Source: CAD feature listing. Evaluate the final solid. Frame: model axes, mm. Face numbers are marked on the shaded views. A direction names the side the tool comes from. Round coordinates to 2 decimals unless told otherwise and drop trailing zeros. Write each loop counter-clockwise with the first axis right and the second up, starting at its lowest first coordinate (ties: lowest second). Pieces come first, ordered by that corner, then holes. Notation, with made-up numbers: M 61.25,31.25 L 104.25,31.25 A17 cw 104.25,64.25 Z; hole C 42,84 d2. An arc over 180 degrees is marked long. Use a Markdown table: item, result.
Autodesk Fusion 360 part; units mm, degrees
sketch "Sketch1" plane through (0, 0, 0) normal (0, 0, 1) x (1, 0, 0)
  line L0 (20.9846, 55.2598) -> (20.9846, 21.2598)
  line L1 (20.9846, 55.2598) -> (24.9846, 55.2598)
  line L2 (24.9846, 55.2598) -> (24.9846, 53.2598)
  line L3 (24.9846, 53.2598) -> (26.9846, 53.2598)
  line L4 (26.9846, 53.2598) -> (26.9846, 57.2598)
  line L5 (26.9846, 57.2598) -> (7.9846, 57.2598)
  line L6 (7.9846, 57.2598) -> (7.9846, 37.2598)
  line L7 (7.9846, 37.2598) -> (18.9846, 37.2598)
  line L8 (18.9846, 37.2598) -> (18.9846, 19.2598)
  line L9 (18.9846, 19.2598) -> (26.485, 19.2598)
  line L10 (20.9846, 21.2598) -> (24.6846, 21.2598)
  line L11 (24.6846, 21.2598) -> (25.485, 22.2598)
  line L12 (25.485, 22.2598) -> (26.485, 22.2598)
  line L13 (26.485, 22.2598) -> (26.485, 19.2598)
  line L14 (9.9846, 55.2598) -> (15.9742, 55.2598)
  line L15 (15.9742, 55.2598) -> (9.9846, 49.9357)
  line L16 (9.9846, 49.9357) -> (9.9846, 55.2598)
  line L17 (9.9846, 44.5839) -> (9.9846, 39.2598)
  line L18 (9.9846, 39.2598) -> (15.9742, 39.2598)
  line L19 (9.9846, 44.5839) -> (15.9742, 39.2598)
  line L20 (9.9846, 47.2598) -> (18.9846, 55.2598)
  line L21 (18.9846, 39.2598) -> (9.9846, 47.2598)
  line L22 (18.9846, 39.2598) -> (18.9846, 55.2598)
  dimension "d1" = 2
  dimension "d2" = 4
  dimension "d3" = 2
  dimension "d4" = 2
  dimension "d5" = 13
  dimension "d6" = 34
  dimension "d7" = 1
  dimension "d8" = 3.7
  dimension "d9" = 1
  dimension "d10" = 2
  dimension "d11" = 20
  dimension "d15" = 2
  dimension "d25" = 2
  dimension "d26" = 2
  dimension "d27" = 2
  dimension "d29" = 2
  dimension "d30" = 2
  dimension "d31" = 2
  dimension "d32" = 2
  dimension "d34" = 2
  dimension "d35" = 2
extrude "Extrude1" add sketch "Sketch1" along normal blind 7.7
fillet "Fillet1" radius 1 9 edges at (7.9846, 37.2598, 3.85) (18.9846, 37.2598, 3.85) (18.9846, 19.2598, 3.85) (26.485, 19.2598, 3.85) (7.9846, 57.2598, 3.85) (26.485, 22.2598, 3.85) (24.9846, 53.2598, 3.85) (26.9846, 53.2598, 3.85) (26.9846, 57.2598, 3.85)
fillet "Fillet1" radius 1 9 edges at (9.9846, 55.2598, 3.85) (15.9742, 55.2598, 3.85) (15.9742, 39.2598, 3.85) (9.9846, 39.2598, 3.85) (20.9846, 38.2598, 7.7) (9.9846, 49.9357, 3.85) (9.9846, 47.2598, 3.85) (18.9846, 55.2598, 3.85) (18.9846, 39.2598, 3.85)
sketch "Sketch2" plane through (0, 57.2598, 0) normal (0, 1, 0) x (-1, 0, 0)
  line L0 (-25.9846, 7.7) -> (-25.9846, 0)
  line L1 (-25.9846, 0) -> (-8.9846, 0)
  line L2 (-8.9846, 0) -> (-8.9846, 7.7)
  line L3 (-8.9846, 7.7) -> (-25.9846, 7.7)
  line L4 (-26.9846, 7.7) -> (-26.9846, 0)
  line L5 (-7.9846, 0) -> (-7.9846, 7.7)
  line L6 (-20.9846, 0) -> (-20.9846, 6.7)
  point P0 (-11.9846, 4)
  point P1 (-20.9846, 0)
  point P2 (-11.9846, 3.7)
  dimension "d16" = 4
  dimension "d22" = 9
  dimension "d23" = 9
  dimension "d24" = 4
hole "Hole1" at (11.9846, 57.2598, 4) at (11.9846, 57.2598, 3.7) direction (0, -1, 0) diameter 5 depth 18 tip angle 160
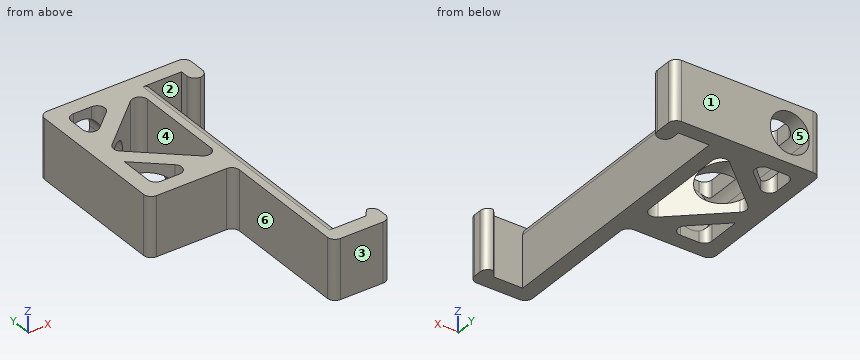
Q1. Section A-A on x = 24. Return loops of the section in (y, z).
Results are:
| item | result |
|---|---|
| outline | M 19.26,0 L 21.26,0 L 21.26,7.7 L 19.26,7.7 Z; M 55.26,0 L 57.26,0 L 57.26,7.7 L 55.26,7.7 Z |
Q2. Line query: L1, parallel to X at y = 53, z = 3; L2, parallel to Y at x = 22.5, z = 3.25; L3, parallel to X at y = 52, z = 0.75. Output: solid intervals per line, ascending.
Results are:
| item | result |
|---|---|
| L1 | 7.98 to 9.58, 14.38 to 16.44, 18.98 to 20.98 |
| L2 | 19.26 to 21.26, 55.26 to 57.26 |
| L3 | 7.98 to 10, 12.31 to 15.32, 18.98 to 20.98 |
Q3. Reachability of the marked faces 4, 5 and 6 from +Z, -Z, +X, -X, +Y, -Y: full face, straight path, thin tool, end or side. Return the list, or none.
Results are:
| item | result |
|---|---|
| face 4 | +Z, -Z |
| face 5 | +Y |
| face 6 | +Z, -Z, -X, -Y |
Q4. Mould query, pull axis Y, two halves, no side actions, for the marked faces 1, 2 and 3. Classes: +Y half, -Y half, draft (parallel to the pull), parting line (faces both ways), or undercut.
Results are:
| item | result |
|---|---|
| face 1 | +Y half |
| face 2 | undercut |
| face 3 | -Y half |
Q5. Section C-C on x = 20.5. Return loops of the section in (y, z).
Results are:
| item | result |
|---|---|
| outline | M 19.26,0 L 57.26,0 L 57.26,7.7 L 55.26,7.7 L 55.26,7.56 L 21.26,7.56 L 21.26,7.7 L 19.26,7.7 Z |
Q6. Section B-B on y = 25. Return loops of the section in (x, z), plus the area to 3 significant figures.
Results are:
| item | result |
|---|---|
| outline | M 18.98,0 L 20.98,0 L 20.98,6.7 A1 ccw 19.98,7.7 L 18.98,7.7 Z |
| area | 15.2 mm^2 |
Q7. First-contact query: pin 1 Ø1.5 at (y, z) = (44, 5.5) entering from +X; pin 2 Ø0.8 at (x, z) = (12, 7) entering from -Y; pin 3 Ø1.7 at (y, z) = (53, 1.5) entering from +X; pin 4 Ø1.5 at (x, y) = (10.5, 36) entering from +Z. Flat tips, straight axial feed; report the tip coordinate or a pass-through.
Results are:
| item | result |
|---|---|
| pin 1 | x = 20.98 |
| pin 2 | y = 37.26 |
| pin 3 | x = 26.9 |
| pin 4 | through |
